Check sheet for the modelled part. Datum: model origin and axes. Units: mm. Face numbers are marked on the shaded views. A direction names the side the tool comes from. Round coordinates to 2 decimals unless told otherwise and drop trailing zeros. Order: outer loops, then holes, each group sorted by start corner. A loop starts at its lowest first (then second) coordinate and runs counter-clockwise, first axis right, second up.
(1) Sectioned sample at B-B, the plane z = -9. Enter the section's corners in (x, y), and give its area (3 significant figures).
(2) Tool access check on the marked faces 5 and 6. Record the directions out of +Z, -Z, +X, -X, +Y, -Y that give a thin tool (end or side, any length) a straight path to the whole face; none if there is none.
(3) Mould release check, pull along Z, two halves, no side actions. Record for the marked faces 1, 2, 3 and 4: released by +Z, released by -Z, zero draft, split by the parting line, or undercut.
(4) Depth check by flat-ended pin: pin 1 (2 mm diameter, centred on x = 7.5, y = 10, fed in from +Z); pin 2 (2 mm diameter, centred on x = 11.5, y = 15.5, fed in from -Z); pin 3 (1 mm diameter, centred on y = -1, z = 8.5, fed in from -X); pin 4 (12 mm diameter, centred on x = 18, z = 6.5, fed in from -Y). Enter the tip coordinate at first touch or a pass-through.
(5) Thickness scan on probe 1 along Y at (x, z) = (1.5, 0); probe 2 along X at (y, z) = (15.5, 9); probe 3 along Y at (x, z) = (7.25, -1.25). Record the ranges inside material, lowest first.
(6) Sectioned sample at D-D, the plane z = 0. Enter the section's corners in (x, y).
(7) Sectioned sample at A-A, the plane y = 7.5. Enter the section's corners in (x, z).
(8) Sectioned sample at C-C, the plane x = 13.5. Enter the section's corners in (y, z), and give its area (3 significant figures).
```python
from build123d import *

# Parameters (mm, degrees)
SKETCH2_W               = 10
SKETCH2_H               = 24
SKETCH2_R               = 1.5
BOSS_EXTRUDE1_DEPTH     = 15
SKETCH3_R               = 6.75
CUT_EXTRUDE1_DEPTH      = 10
SKETCH5_R               = 1
BOSS_EXTRUDE2_DEPTH     = 2
MIRROR2_COPY_1_SKETCH_R = 1
MIRROR2_COPY_1_DEPTH    = 2


with BuildPart() as part:
    # Sketch2 → Boss-Extrude1 (new body)
    with BuildSketch(Plane(origin=(0, 0, 0), x_dir=(1, 0, 0), z_dir=(0, 1, 0))):
        Rectangle(SKETCH2_W, SKETCH2_H)
        with Locations(Location((0, 9, 0), (0, 0, 270))):
            Circle(SKETCH2_R, mode=Mode.SUBTRACT)
        with Locations(Location((0, -9, 0), (0, 0, 90))):
            Circle(SKETCH2_R, mode=Mode.SUBTRACT)
    extrude(amount=BOSS_EXTRUDE1_DEPTH)

    # Sketch3 → Cut-Extrude1 (cut)
    with BuildSketch(Plane(origin=(5, 0, 0), x_dir=(0, 0, -1), z_dir=(1, 0, 0))):
        with Locations((0, 7.5)):
            Circle(SKETCH3_R)
    extrude(amount=-CUT_EXTRUDE1_DEPTH, mode=Mode.SUBTRACT)

    # Sketch5 → Boss-Extrude2 (add)
    with BuildSketch(Plane.XZ):
        with BuildLine():
            Line((0, 0), (0, 2))
            Line((0, 2), (23, 2))
            ThreePointArc((23, 2), (25, 0), (23, -2))
            Line((23, -2), (0, -2))
            Line((0, -2), (0, 0))
        make_face()
        with Locations(Location((23, 0, 0), (0, 0, 270))):
            Circle(SKETCH5_R, mode=Mode.SUBTRACT)
    boss_extrude2 = extrude(amount=BOSS_EXTRUDE2_DEPTH)

    # Mirror1: Boss-Extrude2 across plane
    add(boss_extrude2.mirror(Plane(origin=(0, 7.5, 0), x_dir=(0, 0, 1), z_dir=(0, -1, 0))))

    # Mirror2: Boss-Extrude2 across plane
    add(boss_extrude2.mirror(Plane.XY.offset(4.5)))

    # Mirror2 copy 1 sketch → Mirror2 copy 1 (add)
    with BuildSketch(Plane(origin=(0, 15, 9), x_dir=(1, 0, 0), z_dir=(0, 1, 0))):
        with BuildLine():
            Line((0, 0), (0, 2))
            Line((0, 2), (23, 2))
            ThreePointArc((23, 2), (25, 0), (23, -2))
            Line((23, -2), (0, -2))
            Line((0, -2), (0, 0))
        make_face()
        with Locations(Location((23, 0, 0), (0, 0, 270))):
            Circle(MIRROR2_COPY_1_SKETCH_R, mode=Mode.SUBTRACT)
    extrude(amount=MIRROR2_COPY_1_DEPTH)


solid = part.part
```
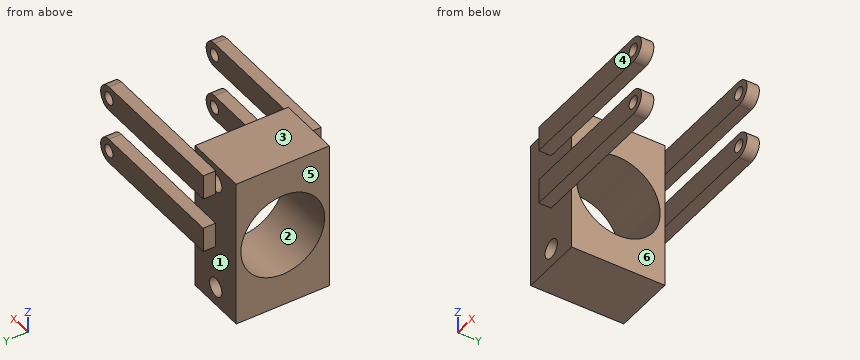
Derived:
1. outline: (-5, 0) - (-1.5, 0) - (-1.5, 15) - (-5, 15) - close; (1.5, 0) - (5, 0) - (5, 15) - (1.5, 15) - close
1. area: 105 mm2
2. face 5: +Z, -Z, -X, +Y, -Y
2. face 6: +Z, -Z, +X
3. face 1: undercut
3. face 2: undercut
3. face 3: released by +Z
3. face 4: zero draft
4. pin 1: passes through
4. pin 2: stops at z = -2
4. pin 3: stops at x = 0
4. pin 4: stops at y = -2
5. probe 1: y = -2 to 0.75, 14.25 to 17
5. probe 2: x = 0 to 22, 24 to 25
5. probe 3: y = -2 to 0, 15 to 17
6. outline: (-5, 0) - (0, 0) - (0, -2) - (22, -2) - (22, 0) - (5, 0) - (5, 0.75) - (-5, 0.75) - close; (-5, 14.25) - (5, 14.25) - (5, 15) - (22, 15) - (22, 17) - (0, 17) - (0, 15) - (-5, 15) - close; (24, -2) - (25, -2) - (25, 0) - (24, 0) - close; (24, 15) - (25, 15) - (25, 17) - (24, 17) - close
7. outline: (-5, -12) - (5, -12) - (5, -6.75) - (-5, -6.75) - close; (-5, 6.75) - (5, 6.75) - (5, 12) - (-5, 12) - close; hole circle Ø3 at (0, -9); hole circle Ø3 at (0, 9)
8. outline: (-2, -2) - (0, -2) - (0, 2) - (-2, 2) - close; (-2, 7) - (0, 7) - (0, 11) - (-2, 11) - close; (15, -2) - (17, -2) - (17, 2) - (15, 2) - close; (15, 7) - (17, 7) - (17, 11) - (15, 11) - close
8. area: 32.0 mm2
